Verification items for the finished model (mm, model axes). Face numbers are marked on the shaded views. A direction names the side the tool comes from. Round coordinates to 2 decimals unless told otherwise and drop trailing zeros. Write each loop counter-clockwise with the first axis right and the second up, starting at its lowest first coordinate (ties: lowest second). Pieces come first, ordered by that corner, then holes. Notation, with made-up numbers: (21, -0.5) - (59, -0.5) arc R28 ccw to (59, 17.5) - close; hole circle Ø4 at (46, -33.5). An arc over 180 degrees is marked (long way). Answer as a JSON object with one key per item and string values. Group by question number.
1) Section check C-C (x = 14). Enter the section's corners in (y, z), then the cut area to 3 significant figures.
2) Set-up check for the marked faces 1, 2 and 3: record each of +Z, -Z, +X, -X, +Y, -Y from which the full face is reachable in a straight line by a thin tool's end or side.
3) Go/stop test with flat-tipped pins: pin 1 Ø1.5 at (x, z) = (-16.5, 2.5) entering from +Y; pin 2 Ø1.5 at (x, z) = (-14.5, 2.5) entering from -Y; pin 3 Ø3 at (x, y) = (0, -1) entering from +Z. Record where each tip stops, or that it passes through.
4) Section check D-D (x = -16). Enter the section's corners in (y, z).
5) Section check B-B (z = -4.5). Enter the section's corners in (x, y).
6) Mould release check, pull along Y, two halves, no side actions. Record for the marked faces 4, 5, 6 and 7: +Y half, -Y half, draft (parallel to the pull), parting line (faces both ways), or undercut.
7) Section check A-A (y = -3.5). Enter the section's corners in (x, z), then the cut area to 4 significant figures.
8) Thickness scan on line 1 (Y direction, x = 11, z = -6.75); line 2 (Z direction, x = -16, y = 2.75); line 3 (X direction, y = -7, z = -2.75). Record the ranges inside material, lowest first.
```python
from build123d import *

# Parameters (mm, degrees)
SKETCH1_W           = 35.6
SKETCH1_H           = 17.8
BOSS_EXTRUDE1_DEPTH = 0.65
SKETCH2_W           = 6
SKETCH2_H           = 8
BOSS_EXTRUDE2_DEPTH = 3
BOSS_EXTRUDE3_DEPTH = 2.5
BOSS_EXTRUDE4_DEPTH = 6.1
CHAMFER1_SIZE       = 0.2


with BuildPart() as part:
    # Sketch1 → Boss-Extrude1 (new, symmetric)
    with BuildSketch(Plane.XY):
        Rectangle(SKETCH1_W, SKETCH1_H)
    extrude(amount=BOSS_EXTRUDE1_DEPTH, both=True)

    # Sketch2 → Boss-Extrude2 (add)
    with BuildSketch(Plane.XY.offset(0.65)):
        with Locations((-15.8, 0)):
            Rectangle(SKETCH2_W, SKETCH2_H)
    extrude(amount=BOSS_EXTRUDE2_DEPTH)

    # Sketch3 → Boss-Extrude3 (add)
    with BuildSketch(Plane(origin=(0, 0, -0.65), x_dir=(-1, 0, 0), z_dir=(0, 0, -1))):
        Polygon((17.8, 6.4), (-15.3, 6.4), (-15.3, -6.4), (17.8, -6.4), (17.8, -8.9), (-17.8, -8.9), (-17.8, 8.9), (17.8, 8.9), align=None)
    extrude(amount=BOSS_EXTRUDE3_DEPTH)

    # Sketch4 → Boss-Extrude4 (add)
    with BuildSketch(Plane(origin=(0, 0, -3.15), x_dir=(-1, 0, 0), z_dir=(0, 0, -1))):
        Polygon((16.85, -7.95), (16.85, -7.35), (-16.25, -7.35), (-16.25, 7.35), (16.85, 7.35), (16.85, 7.95), (-16.85, 7.95), (-16.85, -7.95), align=None)
    extrude(amount=BOSS_EXTRUDE4_DEPTH)

    # Chamfer1
    chamfer1_edges = [part.edges().sort_by_distance(p)[0] for p in [
        (0, -7.95, -9.25),
        (-16.85, -7.65, -9.25),
        (-0.3, -7.35, -9.25),
        (16.25, 0, -9.25),
        (-0.3, 7.35, -9.25),
        (-16.85, 7.65, -9.25),
        (0, 7.95, -9.25),
        (16.85, 0, -9.25),
    ]]
    chamfer(chamfer1_edges, length=CHAMFER1_SIZE)


solid = part.part
```
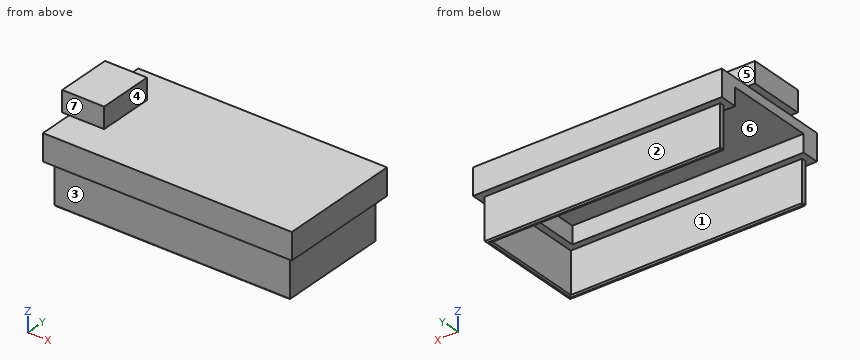
Returned:
{
 "1": {"outline": "(-8.9, -3.15) - (-7.95, -3.15) - (-7.95, -9.05) - (-7.75, -9.25) - (-7.55, -9.25) - (-7.35, -9.05) - (-7.35, -3.15) - (-6.4, -3.15) - (-6.4, -0.65) - (6.4, -0.65) - (6.4, -3.15) - (7.35, -3.15) - (7.35, -9.05) - (7.55, -9.25) - (7.75, -9.25) - (7.95, -9.05) - (7.95, -3.15) - (8.9, -3.15) - (8.9, 0.65) - (-8.9, 0.65) - close", "area": "42.9 mm2"},
 "2": {"face 1": "-Z, -X", "face 2": "-Z, +X, -X, +Y", "face 3": "-Z, +X, -X, -Y"},
 "3": {"pin 1": "y = 4", "pin 2": "y = -4", "pin 3": "z = 0.65"},
 "4": {"outline": "(-8.9, -3.15) - (-7.95, -3.15) - (-7.95, -9.05) - (-7.75, -9.25) - (-7.55, -9.25) - (-7.35, -9.05) - (-7.35, -3.15) - (-6.4, -3.15) - (-6.4, -0.65) - (6.4, -0.65) - (6.4, -3.15) - (7.35, -3.15) - (7.35, -9.05) - (7.55, -9.25) - (7.75, -9.25) - (7.95, -9.05) - (7.95, -3.15) - (8.9, -3.15) - (8.9, 0.65) - (4, 0.65) - (4, 3.65) - (-4, 3.65) - (-4, 0.65) - (-8.9, 0.65) - close"},
 "5": {"outline": "(-16.85, -7.95) - (16.85, -7.95) - (16.85, 7.95) - (-16.85, 7.95) - (-16.85, 7.35) - (16.25, 7.35) - (16.25, -7.35) - (-16.85, -7.35) - close"},
 "6": {"face 4": "draft", "face 5": "+Y half", "face 6": "undercut", "face 7": "-Y half"},
 "7": {"outline": "(-18.8, 0.65) - (-17.8, 0.65) - (-17.8, -0.65) - (15.3, -0.65) - (15.3, -3.15) - (16.25, -3.15) - (16.25, -9.05) - (16.45, -9.25) - (16.65, -9.25) - (16.85, -9.05) - (16.85, -3.15) - (17.8, -3.15) - (17.8, 0.65) - (-12.8, 0.65) - (-12.8, 3.65) - (-18.8, 3.65) - close", "area": "74.15 mm2"},
 "8": {"line 1": "-7.95 to -7.35, 7.35 to 7.95", "line 2": "-0.65 to 3.65", "line 3": "-17.8 to 17.8"}
}
